from build123d import *

# Parameters (mm, degrees)
SKETCH1_W               = 48.5
SKETCH1_H               = 23.5
BOSS_EXTRUDE1_DEPTH     = 12
SHELL1_T                = -1.25
SKETCH2_R               = 4.55
CUT_EXTRUDE1_DEPTH      = 11.75
CUT_EXTRUDE1_DEPTH_BACK = 2.25
SKETCH3_W               = 10.75
SKETCH3_H               = 13
CUT_EXTRUDE2_DEPTH      = 3
CHAMFER1_SIZE           = 1
CUT_EXTRUDE3_REACH      = 25.5
SKETCH5_W               = 5
SKETCH5_H               = 2
SKETCH6_W               = 0.6
SKETCH6_H               = 0.6


with BuildPart() as part:
    # Sketch1 → Boss-Extrude1 (new body)
    with BuildSketch(Plane.XY):
        Rectangle(SKETCH1_W, SKETCH1_H)
    extrude(amount=BOSS_EXTRUDE1_DEPTH)

    # Shell1
    shell1_openings = [part.faces().sort_by_distance(p)[0] for p in [
        (0, 0, 12),
    ]]
    offset(amount=SHELL1_T, openings=shell1_openings, kind=Kind.INTERSECTION)

    # Sketch2 → Cut-Extrude1 (cut, two sides)
    with BuildSketch(Plane.XY.offset(1.25)) as cut_extrude1_sk:
        with Locations((-10.45, 0)):
            Circle(SKETCH2_R)
    extrude(amount=CUT_EXTRUDE1_DEPTH, mode=Mode.SUBTRACT)
    extrude(cut_extrude1_sk.sketch, amount=-CUT_EXTRUDE1_DEPTH_BACK, mode=Mode.SUBTRACT)

    # Sketch3 → Cut-Extrude2 (cut)
    with BuildSketch(Plane(origin=(24.25, 0, 0), x_dir=(0, 0, -1), z_dir=(1, 0, 0))):
        with Locations((-6.625, 0)):
            Rectangle(SKETCH3_W, SKETCH3_H)
    extrude(amount=-CUT_EXTRUDE2_DEPTH, mode=Mode.SUBTRACT)

    # Sweep2: sweep along a curve in space
    with BuildLine() as sweep2_path:
        Line((23, -10.5, 12), (-23, -10.5, 12))
        Line((-23, -10.5, 12), (-23, 10.5, 12))
        Line((-23, 10.5, 12), (23, 10.5, 12))
    # Sketch4 → Sweep2 (sweep)
    with BuildSketch(Plane(origin=(23, 0, 0), x_dir=(0, 0, -1), z_dir=(1, 0, 0))):
        Polygon((-12, -11.75), (-13, -10.75), (-13, -10), (-12, -11), align=None)
    sweep(path=sweep2_path.line, transition=Transition.RIGHT)

    # Chamfer1
    chamfer1_edges = [part.edges().sort_by_distance(p)[0] for p in [
        (0, -11.75, 0),
        (-24.25, 0, 0),
        (0, 11.75, 0),
        (24.25, 0, 0),
        (24.25, -11.75, 6),
        (-24.25, -11.75, 6),
        (-24.25, 11.75, 6),
        (24.25, 11.75, 6),
    ]]
    chamfer(chamfer1_edges, length=CHAMFER1_SIZE)

    # Sketch5 → Cut-Extrude3 (cut, up to next)
    with BuildSketch(Plane(origin=(0, 11.75, 0), x_dir=(1, 0, 0), z_dir=(0, 1, 0)), mode=Mode.PRIVATE) as cut_extrude3_sk1:
        with Locations((14, -6.75)):
            Rectangle(SKETCH5_W, SKETCH5_H)
    cut_extrude3_tool1 = extrude(cut_extrude3_sk1.sketch, amount=-CUT_EXTRUDE3_REACH, mode=Mode.PRIVATE) & part.part
    add(cut_extrude3_tool1.solids().sort_by_distance((14, 11.75, 6.75))[0], mode=Mode.SUBTRACT)

    # Sweep3: sweep along a curve in space
    with BuildLine() as sweep3_path:
        Line((23, -10.5, 12), (-23, -10.5, 12))
        Line((-23, -10.5, 12), (-23, 10.5, 12))
        Line((-23, 10.5, 12), (23, 10.5, 12))
    # Sketch6 → Sweep3 (sweep)
    with BuildSketch(Plane.ZY.offset(-23)):
        with Locations((11.7, -10.2)):
            Rectangle(SKETCH6_W, SKETCH6_H)
    sweep(path=sweep3_path.line, transition=Transition.RIGHT)


solid = part.part
For this review, take the finished solid that the model builds, in its own axes (mm). A direction names the side the tool comes from. Give positions to 0.01 mm unless a question says otherwise; leave off trailing zeros. Order: outer loops, then holes, each group sorted by start corner. A loop starts at its lowest first (then second) coordinate and runs counter-clockwise, first axis right, second up. Notation, with made-up numbers: (-12, -14) - (47, -14) arc R25 ccw to (47, 22) - close; hole circle Ø7 at (69.25, -8). An arc over 180 degrees is marked (long way). Answer as a JSON object with one key per item and string values. Group by question number.
Item 1: Take a section at C-C on z = 7. Give the boundary of the cut face in (x, y), and give its area (3 significant figures).
Item 2: Draft analysis for pull direction X (two halves, no side actions). For faces 1 (the flat face through (-23.74, 0.16, 12.51)), 2 (the flat face through (-0.33, -11.24, 0.49)), 3 (the flat face through (14, 11, 5.75)), state which applies: pulls with the +X half, pulls with the -X half, needs draft (parallel to the pull), parting line crosses it, or undercut.
Item 3: Take a section at B-B on y = 0. Give the boundary of the cut face in (x, z), and give its area (3 significant figures).
Item 4: Wall thickness on line 1 along X through (y, z) = (10.25, 8.5); line 2 along Y through (x, z) = (-18.5, 11.25); line 3 along X through (y, z) = (6.25, 10.75): over which ranges is each line inside the solid? List them lowest first.
Item 5: Take a section at D-D on x = 6. Give the boundary of the cut face in (y, z), and give its area (3 significant figures).
Item 6: Machinability: for faces 4 (the flat face through (-0.1, 10.2, 11.4)), 5 (the flat face through (24, -6.5, 7)), 6 (the flat face through (16.5, 11, 7)), 7 (the flat face through (24, -11, 6)), which of the approach directions +Z, -Z, +X, -X, +Y, -Y give a long, thin tool a straight path to every point of the face, cutting with its end or side? Answer none if there is none.
Item 7: Clearance check with flat-ended pins moving along their axes: pin 1 Ø10.5 at (x, y) = (6, 3.5) entering from +Z; pin 2 Ø5 at (y, z) = (3.5, 6.5) entering from +X. State where each tip first meets the part, or that it passes through.
Item 8: Take a section at A-A on x = 14. Give the boundary of the cut face in (y, z).
Reported:
{
 "1": {"outline": "(-24.25, -10.75) - (-23.25, -11.75) - (23.25, -11.75) - (24.25, -10.75) - (24.25, -6.5) - (23, -6.5) - (23, -10.5) - (-23, -10.5) - (-23, 10.5) - (11.5, 10.5) - (11.5, 11.75) - (-23.25, 11.75) - (-24.25, 10.75) - close; (16.5, 10.5) - (23, 10.5) - (23, 6.5) - (24.25, 6.5) - (24.25, 10.75) - (23.25, 11.75) - (16.5, 11.75) - close", "area": "149 mm^2"},
 "2": {"face 1": "pulls with the -X half", "face 2": "needs draft", "face 3": "undercut"},
 "3": {"outline": "(-24.25, 1) - (-23.25, 0) - (-15, 0) - (-15, 1.25) - (-23, 1.25) - (-23, 11.4) - (-22.4, 11.4) - (-22.4, 12) - (-23.5, 12) - (-22.5, 13) - (-23.25, 13) - (-24.25, 12) - close; (-5.9, 0) - (23.25, 0) - (24.25, 1) - (24.25, 1.25) - (-5.9, 1.25) - close", "area": "62.8 mm^2"},
 "4": {"line 1": "-24.25 to -23, 23 to 24.25", "line 2": "-11.75 to -10.5, 10.5 to 11.75", "line 3": "-24.25 to -23"},
 "5": {"outline": "(-11.75, 1) - (-10.75, 0) - (10.75, 0) - (11.75, 1) - (11.75, 12) - (10.75, 13) - (10, 13) - (11, 12) - (9.9, 12) - (9.9, 11.4) - (10.5, 11.4) - (10.5, 1.25) - (-10.5, 1.25) - (-10.5, 11.4) - (-9.9, 11.4) - (-9.9, 12) - (-11, 12) - (-10, 13) - (-10.75, 13) - (-11.75, 12) - close", "area": "57.5 mm^2"},
 "6": {"face 4": "none", "face 5": "+Z, +X", "face 6": "+Y", "face 7": "+Z, -Z, +X, -Y"},
 "7": {"pin 1": "z = 1.25", "pin 2": "x = -23"},
 "8": {"outline": "(-11.75, 1) - (-10.75, 0) - (10.75, 0) - (11.75, 1) - (11.75, 5.75) - (10.5, 5.75) - (10.5, 1.25) - (-10.5, 1.25) - (-10.5, 11.4) - (-9.9, 11.4) - (-9.9, 12) - (-11, 12) - (-10, 13) - (-10.75, 13) - (-11.75, 12) - close; (9.9, 11.4) - (10.5, 11.4) - (10.5, 7.75) - (11.75, 7.75) - (11.75, 12) - (10.75, 13) - (10, 13) - (11, 12) - (9.9, 12) - close"}
}
